CAD build for the part. Positions are in the model's coordinates, mm. Face numbers are marked on the shaded views. Round coordinates to 2 decimals unless told otherwise and drop trailing zeros. Loops run counter-clockwise (first coordinate to the right, second up) from the corner with the lowest first, then second, coordinate; pieces in that order, holes last.
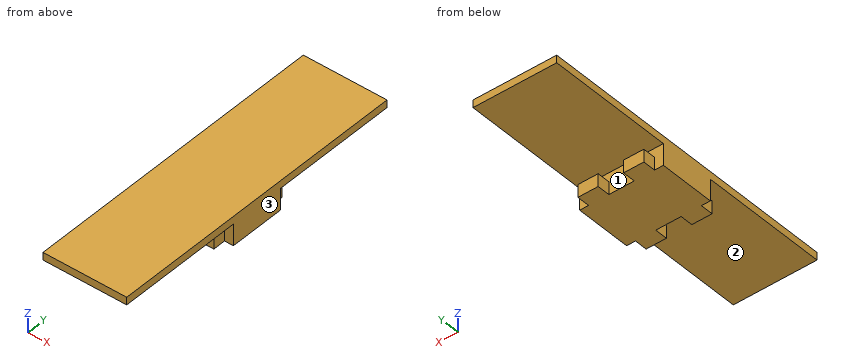
from build123d import *

# Parameters (mm, degrees)
BOSS_EXTRUDE1_DEPTH = 2.5
SKETCH_1_W          = 33
SKETCH_1_H          = 22
EXTRUDE_1_DEPTH     = 6.5
SKETCH_2_W          = 33
SKETCH_2_H          = 3
EXTRUDE_2_DEPTH     = 50


with BuildPart() as part:
    # Sketch1 → Boss-Extrude1 (new, symmetric)
    with BuildSketch(Plane.XY):
        Polygon((-13, 11), (-16.5, 11), (-16.5, -11), (-13, -11), (-13, -16), (-5, -16), (-5, -11), (5, -11), (5, -16), (13, -16), (13, -11), (16.5, -11), (16.5, 11), (13, 11), (13, 16), (5, 16), (5, 11), (-5, 11), (-5, 16), (-13, 16), align=None)
    extrude(amount=BOSS_EXTRUDE1_DEPTH, both=True)

    # 草图1 → 凸台-拉伸1 (add)
    with BuildSketch(Plane.XY.offset(2.5)):
        Rectangle(SKETCH_1_W, SKETCH_1_H)
    extrude(amount=EXTRUDE_1_DEPTH)

    # 草图2 → 凸台-拉伸2 (add)
    with BuildSketch(Plane(origin=(0, 11, 0), x_dir=(1, 0, 0), z_dir=(0, 1, 0))):
        with Locations((0, -7.5)):
            Rectangle(SKETCH_2_W, SKETCH_2_H)
    extrude_2 = extrude(amount=EXTRUDE_2_DEPTH)

    # 镜向1: 凸台-拉伸2 across plane
    add(extrude_2.mirror(Plane.ZX))


solid = part.part
Item 1: Cut at B-B (z = -1). List the corners of the cut face in (x, y).
Verdict:
outline: (-16.5, -11) - (-13, -11) - (-13, -16) - (-5, -16) - (-5, -11) - (5, -11) - (5, -16) - (13, -16) - (13, -11) - (16.5, -11) - (16.5, 11) - (13, 11) - (13, 16) - (5, 16) - (5, 11) - (-5, 11) - (-5, 16) - (-13, 16) - (-13, 11) - (-16.5, 11) - close
Item 2: Mould opens along X. For the marked faces 1, 2 and 3 say: released by +X, released by -X, zero draft, split by the parting line, or undercut.
Verdict:
face 1: undercut
face 2: zero draft
face 3: released by +X
Item 3: Cut at C-C (y = 40.5). List the corners of the cut face in (x, z).
Verdict:
outline: (-16.5, 6) - (16.5, 6) - (16.5, 9) - (-16.5, 9) - close
Item 4: Flat gauge pins, fed straight in: P1, Ø1.5, axis at x = -7.5, z = 0.5, coming from the +Y side; P2, Ø4, axis at y = 13.5, z = 0, coming from the +X side; P3, Ø5.5, axis at x = -8.5, z = -0.5, coming from the -Y side. Where does each tip first touch, or does it go through?
Verdict:
P1: stops at y = 16
P2: stops at x = 13
P3: stops at y = -16
Item 5: Cut at D-D (x = -3). List the corners of the cut face in (y, z).
Verdict:
outline: (-61, 6) - (-11, 6) - (-11, -2.5) - (11, -2.5) - (11, 6) - (61, 6) - (61, 9) - (-61, 9) - close
Item 6: Cut at A-A (x = 10). List the corners of the cut face in (y, z).
Verdict:
outline: (-61, 6) - (-11, 6) - (-11, 2.5) - (-16, 2.5) - (-16, -2.5) - (16, -2.5) - (16, 2.5) - (11, 2.5) - (11, 6) - (61, 6) - (61, 9) - (-61, 9) - close
Item 7: Wall check: L1, parallel to Y at x = 8, z = 1.5; L2, parallel to Y at x = 2, z = 1; L3, parallel to Z at x = 8, y = -28.5. Give the ranges that are in metal, low to high.
Verdict:
L1: y = -16 to 16
L2: y = -11 to 11
L3: z = 6 to 9
